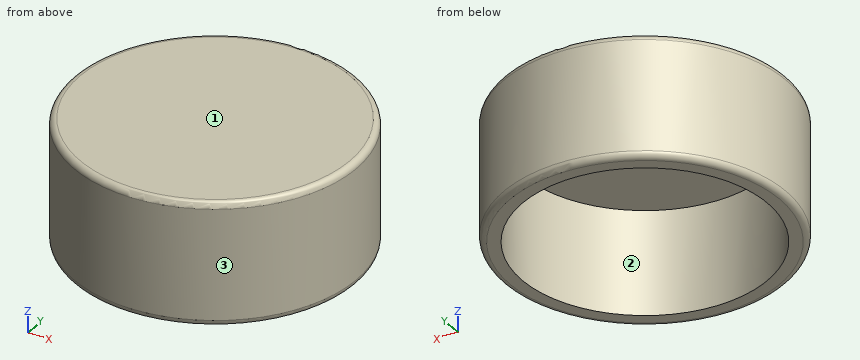
```python
from build123d import *

# Parameters (mm, degrees)
F0_R     = 23
F0_R_2   = 20
F1_DEPTH = 20
F2_R     = 20
F3_DEPTH = 3
F4_R     = 1


with BuildPart() as f1:
    # F0 (on Top) → F1 (new body)
    with BuildSketch(Plane.XY):
        Circle(F0_R)
        Circle(F0_R_2, mode=Mode.SUBTRACT)
    extrude(amount=F1_DEPTH)

    # F2 (on face) → F3 (join)
    with BuildSketch(Plane.XY.offset(20)):
        Circle(F2_R)
    extrude(amount=-F3_DEPTH)

    # F4
    f4_edges = [f1.edges().sort_by_distance(p)[0] for p in [
        (-23, 0, 0),
        (-23, 0, 20),
    ]]
    fillet(f4_edges, radius=F4_R)


solid = f1.part
```
Can you work these out from the model? Positions are in its coordinate system, mm. Face numbers are marked on the shaded views. Coordinates: 2 decimals unless noted, no trailing zeros. Loops run counter-clockwise (first coordinate to the right, second up) from the corner with the lowest first, then second, coordinate; pieces in that order, holes last.
1) Imagine slicing it at C-C on z = 8.75. List the corners of the cut face in (x, y) for me.
2) Imagine slicing it at A-A on x = 0. List the corners of the cut face in (y, z) for me.
3) Thinking about a two-plate mould opening in X: for the marked faces 1, 2 and 3, which applies, pulls with the +X half, pulls with the -X half, needs draft (parallel to the pull), parting line crosses it, or undercut?
4) I need wall thicknesses on probe 1 along Y at (x, z) = (0, 11); probe 2 along Z at (x, y) = (9.5, -0.5); probe 3 along X at (y, z) = (8.5, 15.25). Which ranges of each line are inside material? Lowest first, please.
5) For pin 1 (1.5 mm diameter, centred on x = 14.5, y = 18, fed in from +Z); pin 2 (5 mm diameter, centred on y = 14, z = 11, fed in from +X); pin 3 (8 mm diameter, centred on y = 18.5, z = 6.5, fed in from +X), each with a flat end and sliding along its axis, tell me the tip position at first contact or that it passes through.
Completed:
1. outline: circle Ø46 at (0, 0); hole circle Ø40 at (0, 0)
2. outline: (-23, 1) arc R1 ccw to (-22, 0) - (-20, 0) - (-20, 17) - (20, 17) - (20, 0) - (22, 0) arc R1 ccw to (23, 1) - (23, 19) arc R1 ccw to (22, 20) - (-22, 20) arc R1 ccw to (-23, 19) - close
3. face 1: needs draft
3. face 2: undercut
3. face 3: parting line crosses it
4. probe 1: y = -23 to -20, 20 to 23
4. probe 2: z = 17 to 20
4. probe 3: x = -21.37 to -18.1, 18.1 to 21.37
5. pin 1: stops at z = 19.93
5. pin 2: stops at x = 19.92
5. pin 3: stops at x = 17.85
